Verification items for the finished model (mm, model axes). A direction names the side the tool comes from. Coordinates: 2 decimals unless noted, no trailing zeros. Write each loop counter-clockwise with the first axis right and the second up, starting at its lowest first coordinate (ties: lowest second). Pieces come first, ordered by that corner, then holes. Notation, with made-up numbers: M 50,45 L 94,45 A20 ccw 94,74 Z; hole C -33.75,28.25 d3. An arc over 180 degrees is marked long. Answer in a Markdown table with one row per item.
from build123d import *

# Parameters (mm, degrees)
ESQUISSE1_W          = 2
ESQUISSE1_H          = 3
ESQUISSE1_W_2        = 11.857650871
ESQUISSE1_H_2        = 24
ESQUISSE1_W_3        = 11.857650872
BOSS_EXTRU_1_DEPTH   = 6
D_GAGEMENT_M2_51_D   = 2.5
D_GAGEMENT_M31_D     = 3.25
D_GAGEMENT_M31_DEPTH = 4


with BuildPart() as part:
    # Esquisse1 → Boss.-Extru.1 (new body)
    with BuildSketch(Plane(origin=(0, 0, 0), x_dir=(1, 0, 0), z_dir=(0, 1, 0))):
        Polygon((200.65431579, 26.883578947), (200.65431579, 130.883578947), (76.654558535, 130.883578947), (56.654558535, 157.883578947), (0.654315789, 157.883578947), (0.654315789, -0.116421053), (56.654558535, -0.116421053), (76.654558535, 26.883578947), align=None)
        with Locations((21.225574277, 133.883578948)):
            Rectangle(ESQUISSE1_W, ESQUISSE1_H, mode=Mode.SUBTRACT)
        with Locations((40.083225148, 133.883578948)):
            Rectangle(ESQUISSE1_W, ESQUISSE1_H, mode=Mode.SUBTRACT)
        with Locations((21.225574277, 23.883578948)):
            Rectangle(ESQUISSE1_W, ESQUISSE1_H, mode=Mode.SUBTRACT)
        with Locations((40.083225148, 23.883578948)):
            Rectangle(ESQUISSE1_W, ESQUISSE1_H, mode=Mode.SUBTRACT)
        with Locations((161.22557428, 73.883578947)):
            Rectangle(ESQUISSE1_W, ESQUISSE1_H, mode=Mode.SUBTRACT)
        with Locations((180.083225144, 83.883578947)):
            Rectangle(ESQUISSE1_W, ESQUISSE1_H, mode=Mode.SUBTRACT)
        with Locations((30.654399713, 133.883578948)):
            Rectangle(ESQUISSE1_W_2, ESQUISSE1_H_2, mode=Mode.SUBTRACT)
        with Locations((30.654399713, 23.883578948)):
            Rectangle(ESQUISSE1_W_2, ESQUISSE1_H_2, mode=Mode.SUBTRACT)
        with Locations((170.654399716, 78.883578947)):
            Rectangle(ESQUISSE1_W_3, ESQUISSE1_H_2, mode=Mode.SUBTRACT)
        with Locations((180.083225144, 73.883578947)):
            Rectangle(ESQUISSE1_W, ESQUISSE1_H, mode=Mode.SUBTRACT)
        with Locations((161.22557428, 83.883578947)):
            Rectangle(ESQUISSE1_W, ESQUISSE1_H, mode=Mode.SUBTRACT)
    extrude(amount=BOSS_EXTRU_1_DEPTH)

    # Dégagement M2.51 (through all)
    with Locations(Plane(origin=(0, 6, 0), x_dir=(1, 0, 0), z_dir=(0, 1, 0))):
        with Locations((9.654315789, 148.883578947), (9.654315789, 8.883578947), (76.654315789, 78.883578947), (94.65431579, 78.883578947), (191.65431579, 78.883578947)):
            Hole(D_GAGEMENT_M2_51_D / 2)

    # Dégagement M31
    with Locations(Plane(origin=(0, 0, 0), x_dir=(-1, 0, 0), z_dir=(0, -1, 0))):
        with Locations((-191.65431579, 78.883578947), (-9.654315789, 8.883578947), (-9.654315789, 148.883578947)):
            Hole(D_GAGEMENT_M31_D / 2, depth=D_GAGEMENT_M31_DEPTH)


solid = part.part
1) Sectioned sample at A-A (z = -128.5). Record the cut outline in (x, y).
Response values:
| item | result |
|---|---|
| outline | M 0.65,0 L 24.73,0 L 24.73,6 L 0.65,6 Z; M 36.58,0 L 200.65,0 L 200.65,6 L 36.58,6 Z |
2) Sectioned sample at B-B (x = 30.5). Record the cut outline in (y, z).
Response values:
| item | result |
|---|---|
| outline | M 0,-157.88 L 6,-157.88 L 6,-145.88 L 0,-145.88 Z; M 0,-121.88 L 6,-121.88 L 6,-35.88 L 0,-35.88 Z; M 0,-11.88 L 6,-11.88 L 6,0.12 L 0,0.12 Z |
3) Release check for a two-part mould opening along X. For faces 6 (the face through (99, 6, -80)), 7 (the face through (200.654, 3, -78)), 8 (the face through (36.583, 3, -24)) record: +X half, -X half, draft (parallel to the pull), parting line (faces both ways), or undercut.
Response values:
| item | result |
|---|---|
| face 6 | draft |
| face 7 | +X half |
| face 8 | undercut |
4) Sectioned sample at C-C (y = 0.9). Give the number of separate pieces and of enclosed holes in the cut face, then the cut area to 3 significant figures.
Response values:
| item | result |
|---|---|
| separate pieces | 1 |
| enclosed holes | 16 |
| area | 23,400 mm² |
5) Sectioned sample at D-D (x = 109). Record the cut outline in (y, z), then the cut area to 3 significant figures.
Response values:
| item | result |
|---|---|
| outline | M 0,-130.88 L 6,-130.88 L 6,-26.88 L 0,-26.88 Z |
| area | 624 mm² |
6) Tool access check on faces 1 (the face through (140, 3, -130.884)), 2 (the face through (28, 3, 0.116)), 3 (the face through (171, 3, -66.884)), 4 (the face through (138, 3, -26.884)), 5 (the face through (99, 0, -80)). Record the directions out of +Z, -Z, +X, -X, +Y, -Y that give a thin tool (end or side, any length) a straight path to the whole face; none if there is none.
Response values:
| item | result |
|---|---|
| face 1 | -Z, +X, +Y, -Y |
| face 2 | +Z, +X, -X, +Y, -Y |
| face 3 | +Y, -Y |
| face 4 | +Z, +X, +Y, -Y |
| face 5 | +Z, -Z, +X, -X, -Y |
7) Depth check by flat-ended pin: pin 1 (1 mm diameter, centred on x = 77, y = 2.5, fed in from -Z); pin 2 (5 mm diameter, centred on x = 93, z = -35, fed in from -Y); pin 3 (1 mm diameter, centred on x = 161, y = 2.5, fed in from +Z); pin 4 (1.5 mm diameter, centred on y = 3, z = -134, fed in from +X). Enter the tip coordinate at first touch or a pass-through.
Response values:
| item | result |
|---|---|
| pin 1 | stops at z = -131.09 |
| pin 2 | stops at y = 0 |
| pin 3 | stops at z = -26.88 |
| pin 4 | stops at x = 74.9 |
8) Thickness scan on L1, parallel to Z at x = 28.5, y = 3.95; L2, parallel to Z at x = 21, y = 3.05; L3, parallel to X at y = 0.95, z = -126. Record the ranges inside material, lowest first. Write a range as [from, to].
Response values:
| item | result |
|---|---|
| L1 | z = [-157.88, -145.88], [-121.88, -35.88], [-11.88, 0.12] |
| L2 | z = [-157.88, -135.38], [-132.38, -25.38], [-22.38, 0.12] |
| L3 | x = [0.65, 24.73], [36.58, 200.65] |
